```python
from build123d import *

# Parameters (mm, degrees)
SKETCH1_W           = 57
SKETCH1_H           = 87
BOSS_EXTRUDE1_DEPTH = 5
BOSS_EXTRUDE2_DEPTH = 5
BOSS_EXTRUDE3_START = -87
BOSS_EXTRUDE3_DEPTH = 5


with BuildPart() as part:
    # Sketch1 → Boss-Extrude1 (new body)
    with BuildSketch(Plane(origin=(0, 0, 0), x_dir=(1, 0, 0), z_dir=(0, 1, 0))):
        Rectangle(SKETCH1_W, SKETCH1_H)
    extrude(amount=BOSS_EXTRUDE1_DEPTH)

    # Sketch2 → Boss-Extrude2 (add)
    with BuildSketch(Plane.XY.offset(43.5)):
        Polygon((3.333333333, 0), (-3.333333333, 0), (-5, -2.886751346), (5, -2.886751346), align=None)
    extrude(amount=-BOSS_EXTRUDE2_DEPTH)

    # Sketch2<3> → Boss-Extrude3 (add)
    with BuildSketch(Plane.XY.offset(43.5).offset(BOSS_EXTRUDE3_START)):
        Polygon((3.333333333, 0), (-3.333333333, 0), (-5, -2.886751346), (5, -2.886751346), align=None)
    extrude(amount=BOSS_EXTRUDE3_DEPTH)


solid = part.part
```
Geometry: final body of the model. Coordinates: model frame, mm. A direction names the side the tool comes from. Round coordinates to 2 decimals unless told otherwise and drop trailing zeros. Loops run counter-clockwise (first coordinate to the right, second up) from the corner with the lowest first, then second, coordinate; pieces in that order, holes last. Notation, with made-up numbers: (-17, -17) -> (0, -17) arc R12 cw to (0, -8) -> close; hole circle Ø9 at (48.25, 54.25). An arc over 180 degrees is marked (long way). Use one line per item in the form item = value. Start each with the question number.
1) First-contact query: P1, Ø1.5, axis at x = -4.5, z = 4, coming from the -Y side. Flat tip, straight axial feed; report the tip coordinate or a pass-through.
2) Line query: L1, parallel to Z at x = 0, y = -1.25; L2, parallel to Y at x = -6.5, z = 37. Output: solid intervals per line, ascending.
3) Section A-A on y = -1.25. Output: boundary loops of the cut face in (x, z), then the cut area to 3 significant figures.
4) Draft query along Y for faces 3 (the flat face through (-4.155, -1.423, -41.035)), 4 (the flat face through (4.2, -1.5, 41)), 5 (the flat face through (0, 2, -43.5)), 6 (the flat face through (0, 5, -1)). Return one class per face: released by +Y, released by -Y, zero draft, split by the parting line, or undercut.
5) Section C-C on z = 31.5. Output: boundary loops of the cut face in (x, y).
6) Section B-B on x = -11. Output: boundary loops of the cut face in (y, z).
7) Access query for faces 1 (the flat face through (-28.5, 2, 1)), 2 (the flat face through (0, -1, -38.5)). Directions: +Z, -Z, +X, -X, +Y, -Y. A direction counts if a zero-diameter tool reaches every point of the face in a straight line with its end or side. Return the directions, or none.
Response:
q1.P1 = 0
q2.L1 = -43.5 to -38.5, 38.5 to 43.5
q2.L2 = 0 to 5
q3.outline = (-4.06, -43.5) -> (4.06, -43.5) -> (4.06, -38.5) -> (-4.06, -38.5) -> close; (-4.06, 38.5) -> (4.06, 38.5) -> (4.06, 43.5) -> (-4.06, 43.5) -> close
q3.area = 81.1 mm^2
q4.face_3 = undercut
q4.face_4 = undercut
q4.face_5 = zero draft
q4.face_6 = released by +Y
q5.outline = (-28.5, 0) -> (28.5, 0) -> (28.5, 5) -> (-28.5, 5) -> close
q6.outline = (0, -43.5) -> (5, -43.5) -> (5, 43.5) -> (0, 43.5) -> close
q7.face_1 = +Z, -Z, -X, +Y, -Y
q7.face_2 = +X, -X, -Y
